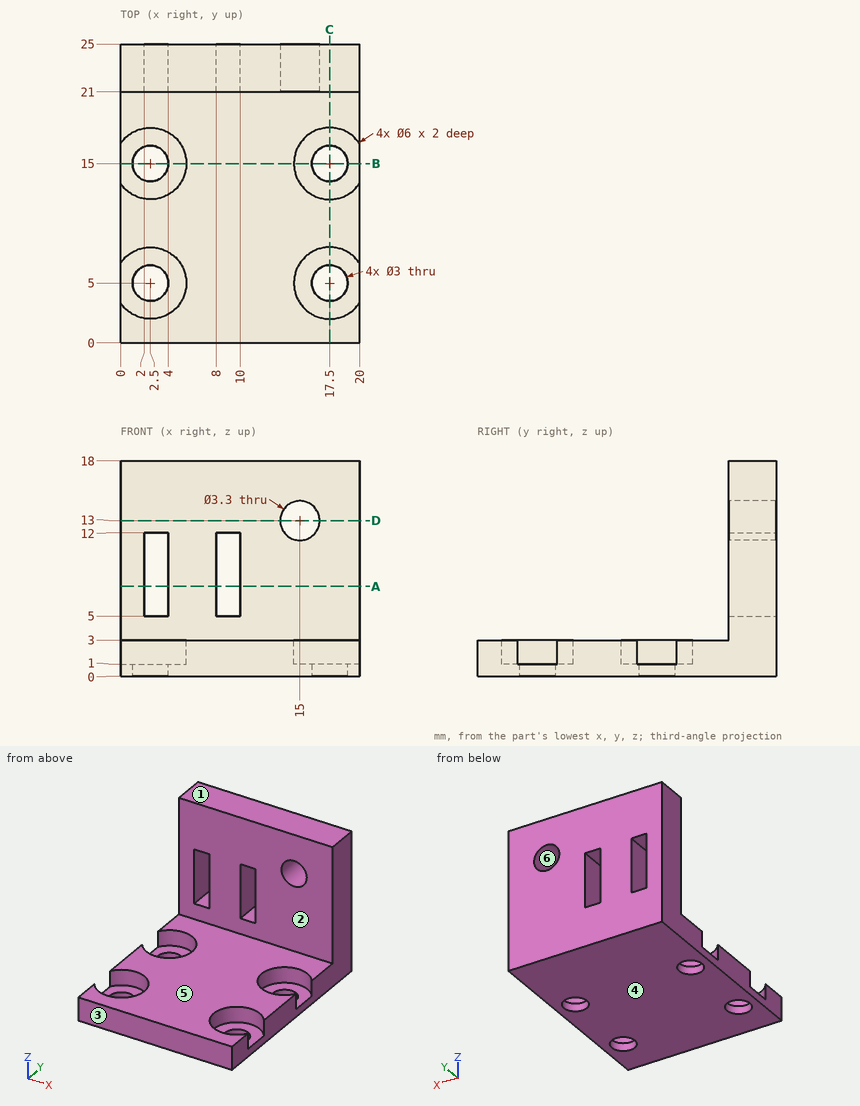
For this review, use the dimensioned drawing (mm, ordinates from the lowest corner) and the shaded views. A direction names the side the tool comes from. Coordinates: 2 decimals unless noted, no trailing zeros. Write each loop counter-clockwise with the first axis right and the second up, starting at its lowest first coordinate (ties: lowest second). Pieces come first, ordered by that corner, then holes. Notation, with made-up numbers: (-10.75, -2.75) - (38.25, -2.75) arc R10 ccw to (38.25, 7.25) - close; hole circle Ø9 at (62, 14). An arc over 180 degrees is marked (long way). Answer as a JSON object with one key per item and string values. Group by question number.
1. To check wall thickness, follow probe 1 along Y at (x, z) = (2.5, 1.9); probe 2 along Y at (x, z) = (2.5, 0.5); probe 3 along X at (y, z) = (5, 0.7). State the ranges of each line that lie inside material, in increasing order.
2. Clearance check with flat-ended pins moving along their axes: pin 1 Ø1 at (y, z) = (20, 6.5) entering from -X; pin 2 Ø3.5 at (x, y) = (17.5, 5) entering from +Z; pin 3 Ø4 at (y, z) = (10, 4.5) entering from -X; pin 4 Ø10 at (x, y) = (10, 13.5) entering from +Z. State where each tip first meets the part, or that it passes through.
3. Add section C-C (x = 17.5). Give the boundary of the cut face in (y, z).
4. Add section D-D (z = 13). Give the boundary of the cut face in (x, y).
5. Add section A-A (z = 7.5). Give the boundary of the cut face in (x, y), plus the area to 3 significant figures.
6. Mouldability with a two-part tool opening along Z and no side actions: class the marked faces 3, 4, 5 and 6 as pulls with the +Z half, pulls with the -Z half, needs draft (parallel to the pull), parting line crosses it, or undercut.
7. Machinability: for the marked faces 1 and 2, which of the approach directions +Z, -Z, +X, -X, +Y, -Y give a long, thin tool a straight path to every point of the face, cutting with its end or side? Answer none if there is none.
8. Add section B-B (y = 15). Give the boundary of the cut face in (x, z).
Findings:
{
 "1": {"probe 1": "0 to 2, 8 to 12, 18 to 25", "probe 2": "0 to 3.5, 6.5 to 13.5, 16.5 to 25", "probe 3": "0 to 1, 4 to 16, 19 to 20"},
 "2": {"pin 1": "through", "pin 2": "z = 1", "pin 3": "x = 0", "pin 4": "z = 3"},
 "3": {"outline": "(0, 0) - (3.5, 0) - (3.5, 1) - (2, 1) - (2, 3) - (0, 3) - close; (6.5, 0) - (13.5, 0) - (13.5, 1) - (12, 1) - (12, 3) - (8, 3) - (8, 1) - (6.5, 1) - close; (16.5, 0) - (25, 0) - (25, 18) - (21, 18) - (21, 3) - (18, 3) - (18, 1) - (16.5, 1) - close"},
 "4": {"outline": "(0, 21) - (13.35, 21) - (13.35, 25) - (0, 25) - close; (16.65, 21) - (20, 21) - (20, 25) - (16.65, 25) - close"},
 "5": {"outline": "(0, 21) - (2, 21) - (2, 25) - (0, 25) - close; (4, 21) - (8, 21) - (8, 25) - (4, 25) - close; (10, 21) - (20, 21) - (20, 25) - (10, 25) - close", "area": "64.0 mm²"},
 "6": {"face 3": "needs draft", "face 4": "pulls with the -Z half", "face 5": "pulls with the +Z half", "face 6": "undercut"},
 "7": {"face 1": "+Z, +X, -X, +Y, -Y", "face 2": "+Z, +X, -X, -Y"},
 "8": {"outline": "(0, 0) - (1, 0) - (1, 1) - (0, 1) - close; (4, 0) - (16, 0) - (16, 1) - (14.5, 1) - (14.5, 3) - (5.5, 3) - (5.5, 1) - (4, 1) - close; (19, 0) - (20, 0) - (20, 1) - (19, 1) - close"}
}
